The model under review builds one solid part; all positions refer to its coordinate system, in mm. A direction names the side the tool comes from. Coordinates: 2 decimals unless noted, no trailing zeros. Loops run counter-clockwise (first coordinate to the right, second up) from the corner with the lowest first, then second, coordinate; pieces in that order, holes last. Notation, with made-up numbers: (35, -8.5) - (55, -8.5) arc R24 cw to (55, 28.5) - close; hole circle Ø1 at (72.25, -39). An arc over 180 degrees is marked (long way). Use a Markdown table: item, result. Add a question column.
1) The part is to be moulded in two halves that separate along X. For faces 1 (the flat face through (35, 26, -13)), 2 (the cylindrical face through (26.968, 25.628, -7.403)), 3 (the flat face through (17.255, 57.552, -16.406)), say which applies: pulls with the +X half, pulls with the -X half, needs draft (parallel to the pull), parting line crosses it, or undercut.
2) Add section B-B, the plane x = 6.5. Give the boundary of the cut face in (y, z), and give its area (3 significant figures).
3) For faces 4 (the cylindrical face through (5, 2.2, -5.8)), 5 (the flat face through (4.6, 4.5, -21.9)), list the 3-axis set-ups (+Z, -Z, +X, -X, +Y, -Y) from which the entire face can be reached by the end or side of a thin tool; tool diameter is ignored.
4) To check wall thickness, follow L1, parallel to X at y = 29.5, z = -5; L2, parallel to Z at x = 28.5, y = 22; L3, parallel to X at y = 3.2, z = -5. State the ranges of each line that lie inside material, in increasing order. Write a range as [from, to].
5) Add section D-D, the plane x = 14.5. Give the boundary of the cut face in (y, z), and give its area (3 significant figures).
6) Add section A-A, the plane y = 36. Give the boundary of the cut face in (x, z).
7) Clearance check with flat-ended pins moving along their axes: pin 1 (6.5 mm diameter, centred on x = 5.5, z = -4, fed in from +Y); pin 2 (4.5 mm diameter, centred on x = 28.5, z = -5, fed in from +Y); pin 3 (1.5 mm diameter, centred on x = 26.5, z = -6.5, fed in from +Y). State where each tip first meets the part, or that it passes through.
8) Add section C-C, the plane z = -21. Give the boundary of the cut face in (x, y).
```python
from build123d import *

# Parameters (mm, degrees)
AUFSATZ_LINEAR_AUSTRAGEN1_DEPTH      = 35
SKIZZE3_R                            = 6
AUFSATZ_LINEAR_AUSTRAGEN2_DEPTH      = 5
SKIZZE4_R                            = 6.5
AUFSATZ_LINEAR_AUSTRAGEN3_DEPTH      = 0.1
SKIZZE7_R                            = 2.85
SCHNITT_LINEAR_AUSTRAGEN1_DEPTH      = 61.311555509
F_3_4_3_4_DURCHMESSER_BOHRUNG1_D     = 3.4
F_3_4_3_4_DURCHMESSER_BOHRUNG1_DEPTH = 4.5


with BuildPart() as part:
    # Skizze1 → Aufsatz-Linear austragen1 (new body)
    with BuildSketch(Plane(origin=(0, 0, 0), x_dir=(0, 0, -1), z_dir=(1, 0, 0))):
        Polygon((0, 0), (22.497566339, 0), (26.82, 0), (26.82, 64.811555509), (22.497566339, 64.811555509), (0, 38), align=None)
    extrude(amount=AUFSATZ_LINEAR_AUSTRAGEN1_DEPTH)

    # Skizze3 → Aufsatz-Linear austragen2 (add)
    with BuildSketch(Plane(origin=(0, 15.700684624, 18.711347307), x_dir=(1, 0, 0), z_dir=(0, 0.64278761, 0.766044443))):
        with Locations((17.5, 46.609688839)):
            Circle(SKIZZE3_R)
    extrude(amount=AUFSATZ_LINEAR_AUSTRAGEN2_DEPTH)

    # Skizze4 → Aufsatz-Linear austragen3 (add)
    with BuildSketch(Plane(origin=(0, 15.700684624, 18.711347307), x_dir=(1, 0, 0), z_dir=(0, 0.64278761, 0.766044443))):
        with Locations((17.5, 46.609688839)):
            Circle(SKIZZE4_R)
    extrude(amount=AUFSATZ_LINEAR_AUSTRAGEN3_DEPTH)

    # Skizze7 → Schnitt-Linear austragen1 (cut, through all)
    with BuildSketch(Plane(origin=(0, 4.5, 0), x_dir=(-1, 0, 0), z_dir=(0, -1, 0))):
        with Locations((-28.5, 5)):
            Circle(SKIZZE7_R)
        with Locations((-6.5, 5)):
            Circle(SKIZZE7_R)
        with Locations((-6.5, 21.82)):
            Circle(SKIZZE7_R)
        with Locations((-28.5, 21.82)):
            Circle(SKIZZE7_R)
    extrude(amount=-SCHNITT_LINEAR_AUSTRAGEN1_DEPTH, mode=Mode.SUBTRACT)

    # Ø3.4 (3.4) Durchmesser Bohrung1
    with Locations(Plane(origin=(6.5, 4.5, -5), x_dir=(0, 0, 1), z_dir=(0, 1, 0))):
        with Locations((0, 0), (-16.82, 0), (-16.82, 22), (0, 22)):
            Hole(F_3_4_3_4_DURCHMESSER_BOHRUNG1_D / 2, depth=F_3_4_3_4_DURCHMESSER_BOHRUNG1_DEPTH)


solid = part.part
```
From the geometry:
| question | item | result |
|---|---|---|
| 1 | face 1 | pulls with the +X half |
| 1 | face 2 | undercut |
| 1 | face 3 | needs draft |
| 2 | outline | (0, -26.82) - (64.81, -26.82) - (64.81, -24.67) - (4.5, -24.67) - (4.5, -23.52) - (0, -23.52) - close; (0, -20.12) - (4.5, -20.12) - (4.5, -18.97) - (60.61, -18.97) - (47.36, -7.85) - (4.5, -7.85) - (4.5, -6.7) - (0, -6.7) - close; (0, -3.3) - (4.5, -3.3) - (4.5, -2.15) - (40.56, -2.15) - (38, 0) - (0, 0) - close |
| 2 | area | 845 mm^2 |
| 3 | face 4 | +Y, -Y |
| 3 | face 5 | +Y |
| 4 | L1 | x = [0, 3.65], [9.35, 25.65], [31.35, 35] |
| 4 | L2 | z = [-26.82, -24.67], [-18.97, -7.85], [-2.15, 0] |
| 4 | L3 | x = [0, 4.8], [8.2, 26.8], [30.2, 35] |
| 5 | outline | (0, -26.82) - (64.81, -26.82) - (64.81, -22.5) - (55.82, -14.96) - (55.89, -14.88) - (55.45, -14.51) - (58.6, -10.76) - (50.64, -4.08) - (47.49, -7.83) - (47.05, -7.47) - (46.99, -7.54) - (38, 0) - (0, 0) - close |
| 5 | area | 1,490 mm^2 |
| 6 | outline | (0, -26.82) - (35, -26.82) - (35, 0) - (0, 0) - close; hole circle Ø5.7 at (6.5, -21.82); hole circle Ø5.7 at (6.5, -5); hole circle Ø5.7 at (28.5, -21.82); hole circle Ø5.7 at (28.5, -5) |
| 7 | pin 1 | stops at y = 46.49 |
| 7 | pin 2 | stops at y = 4.5 |
| 7 | pin 3 | stops at y = 46.64 |
| 8 | outline | (0, 0) - (5.01, 0) - (5.01, 4.5) - (3.77, 4.5) - (3.77, 63.03) - (0, 63.03) - close; (7.99, 0) - (27.01, 0) - (27.01, 4.5) - (25.77, 4.5) - (25.77, 63.03) - (9.23, 63.03) - (9.23, 4.5) - (7.99, 4.5) - close; (29.99, 0) - (35, 0) - (35, 63.03) - (31.23, 63.03) - (31.23, 4.5) - (29.99, 4.5) - close |
